Part print with two shaded views. Sizes in mm from the minimum x, y, z corner. A direction names the side the tool comes from. Round coordinates to 2 decimals unless told otherwise and drop trailing zeros. Write each loop counter-clockwise with the first axis right and the second up, starting at its lowest first coordinate (ties: lowest second). Pieces come first, ordered by that corner, then holes. Notation, with made-up numbers: M 82.25,1 L 135.25,1 A27 cw 135.25,23 Z; hole C -19.5,58 d4. An arc over 180 degrees is marked long. One line per question, with ' | ' between items. Start each with the question number.
1) Mould opens along X. For the marked faces 3, 4 and 5 say: pulls with the +X half, pulls with the -X half, needs draft (parallel to the pull), parting line crosses it, or undercut.
2) Tool access for the marked faces 1 and 2: list every direction of +Z, -Z, +X, -X, +Y, -Y with a clear straight run to the whole face (end or side of a thin tool).
3) Saw through at A-A (y = 15). List the corners of the cut face in (x, z), plus the area to 3 significant figures.
4) Drop flat-ended pins along their axis: pin 1 Ø2 at (x, z) = (19, 3.5) entering from +Y; pin 2 Ø3 at (x, y) = (17.5, 10.5) entering from +Z; pin 3 Ø3 at (x, y) = (23, 19.5) entering from +Z. Give the stop position or say it passes through.
5) Saw through at D-D (z = 8.5). List the corners of the cut face in (x, y), plus the area to 3 significant figures.
6) Wall check: probe 1 along Y at (x, z) = (15, 20.4); probe 2 along Y at (x, z) = (15, 12); probe 3 along Z at (x, y) = (12.75, 15.25). Give the ranges that are in metal, low to high. Write a range as [from, to].
7) Saw through at C-C (z = 20.5). List the corners of the cut face in (x, y), plus the area to 3 significant figures.
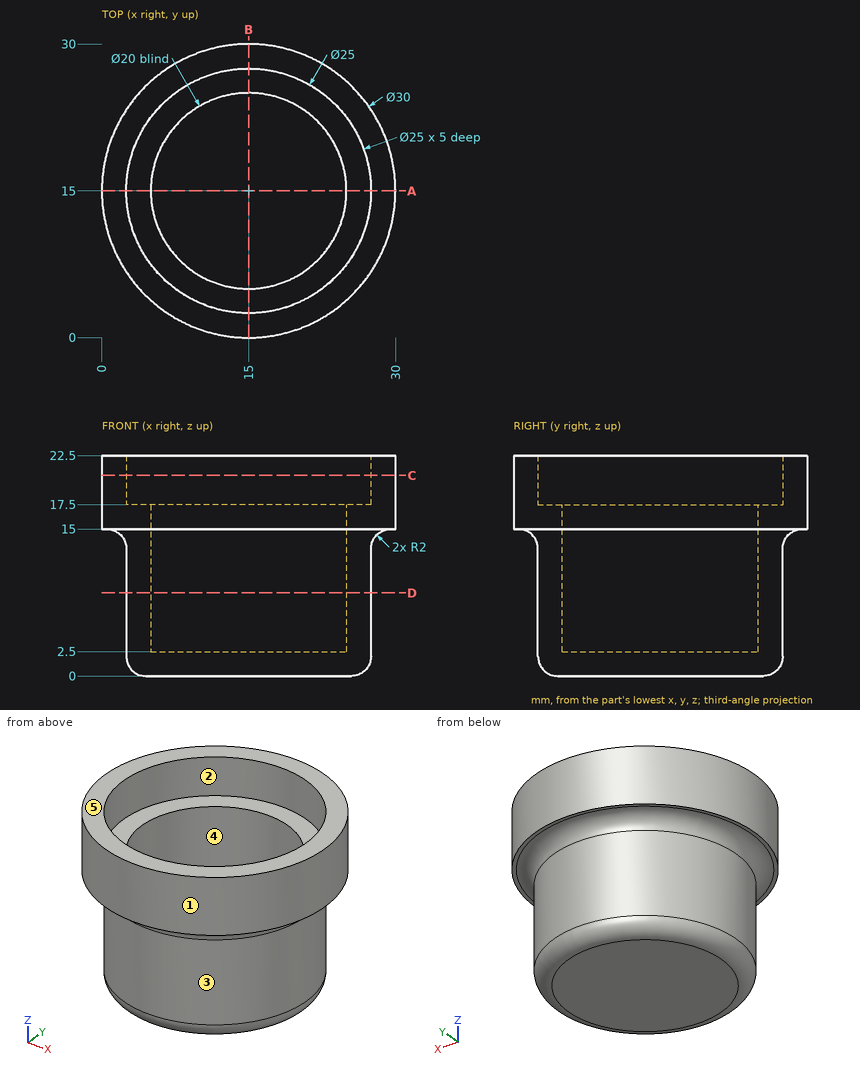
Answer key:
1) face 3: parting line crosses it | face 4: undercut | face 5: needs draft
2) face 1: +Z, -Z | face 2: +Z
3) outline: M 0,15 L 0.5,15 A2 cw 2.5,13 L 2.5,2 A2 ccw 4.5,0 L 25.5,0 A2 ccw 27.5,2 L 27.5,13 A2 cw 29.5,15 L 30,15 L 30,22.5 L 27.5,22.5 L 27.5,17.5 L 25,17.5 L 25,2.5 L 5,2.5 L 5,17.5 L 2.5,17.5 L 2.5,22.5 L 0,22.5 Z | area: 175 mm2
4) pin 1: stops at y = 27.13 | pin 2: stops at z = 2.5 | pin 3: stops at z = 17.5
5) outline: C 15,15 d25; hole C 15,15 d20 | area: 177 mm2
6) probe 1: y = [0, 2.5], [27.5, 30] | probe 2: y = [2.5, 5], [25, 27.5] | probe 3: z = [0, 2.5]
7) outline: C 15,15 d30; hole C 15,15 d25 | area: 216 mm2
